Could you check a few things on this model? Use its own coordinates, in mm. A direction names the side the tool comes from. Round coordinates to 2 decimals unless told otherwise and drop trailing zeros. Loops run counter-clockwise (first coordinate to the right, second up) from the corner with the lowest first, then second, coordinate; pieces in that order, holes last. Notation, with made-up numbers: M 5,67.25 L 32,67.25 A22 cw 32,76.25 Z; hole C 82,-2.5 d6. An arc over 180 degrees is marked long. Answer in a Markdown table with one row per item.
```python
from build123d import *

# Parameters (mm, degrees)
SKETCH3_W           = 70
SKETCH3_H           = 70
BOSS_EXTRUDE1_DEPTH = 2.105
SKETCH6_R           = 3
SKETCH6_W           = 30
SKETCH6_H           = 30
CUT_EXTRUDE5_DEPTH  = 2.105
CUT_EXTRUDE7_DEPTH  = 0.2
FILLET1_R           = 3


with BuildPart() as part:
    # Sketch3 → Boss-Extrude1 (new body)
    with BuildSketch(Plane.XY):
        Rectangle(SKETCH3_W, SKETCH3_H)
    extrude(amount=BOSS_EXTRUDE1_DEPTH)

    # Sketch6 → Cut-Extrude5 (cut)
    with BuildSketch(Plane.XY.offset(2.105)):
        with Locations((0, 25)):
            Circle(SKETCH6_R)
        with Locations((25, 25)):
            Circle(SKETCH6_R)
        with Locations((25, 0)):
            Circle(SKETCH6_R)
        with Locations((25, -25)):
            Circle(SKETCH6_R)
        with Locations((0, -25)):
            Circle(SKETCH6_R)
        with Locations((-25, -25)):
            Circle(SKETCH6_R)
        with Locations((-25, 0)):
            Circle(SKETCH6_R)
        with Locations((-25, 25)):
            Circle(SKETCH6_R)
        Rectangle(SKETCH6_W, SKETCH6_H)
    extrude(amount=-CUT_EXTRUDE5_DEPTH, mode=Mode.SUBTRACT)

    # Sketch8 → Cut-Extrude7 (cut)
    with BuildSketch(Plane.XY.offset(2.105)):
        with BuildLine():
            Line((15, 5), (15, 15))
            Line((15, 15), (20.732380758, 13.932380758))
            ThreePointArc((20.732380758, 13.932380758), (24, 10), (20.732380758, 6.067619242))
            Line((20.732380758, 6.067619242), (15, 5))
        make_face()
        with BuildLine():
            Line((-15, -15), (-20.732380758, -13.932380758))
            ThreePointArc((-20.732380758, -13.932380758), (-24, -10), (-20.732380758, -6.067619242))
            Line((-20.732380758, -6.067619242), (-15, -5))
            Line((-15, -5), (-15, -15))
        make_face()
    extrude(amount=-CUT_EXTRUDE7_DEPTH, mode=Mode.SUBTRACT)

    # Fillet1
    fillet1_edges = [part.edges().sort_by_distance(p)[0] for p in [
        (35, -35, 1.0525),
        (-35, -35, 1.0525),
        (-35, 35, 1.0525),
        (35, 35, 1.0525),
    ]]
    fillet(fillet1_edges, radius=FILLET1_R)


solid = part.part
```
1) If we mould it in two halves opening along Y, with no side actions, what happens to faces 4 (the face through (34.1, -34.14, 1.07)), 5 (the face through (34.1, 34.14, 1.07)), 6 (the face through (22, 0, 1)), 7 (the face through (-0.65, -27.93, 1.07))? For each: released by +Y, released by -Y, zero draft, split by the parting line, or undercut.
Computed:
| item | result |
|---|---|
| face 4 | released by -Y |
| face 5 | released by +Y |
| face 6 | undercut |
| face 7 | undercut |
2) I want a section at A-A, the plane x = -25. Please give me the cut outline in (y, z) (3 decimals), plus the area to 3 significant figures.
Computed:
| item | result |
|---|---|
| outline | M -35,0 L -28,0 L -28,2.105 L -35,2.105 Z; M -22,0 L -3,0 L -3,2.105 L -22,2.105 Z; M 3,0 L 22,0 L 22,2.105 L 3,2.105 Z; M 28,0 L 35,0 L 35,2.105 L 28,2.105 Z |
| area | 109 mm² |
3) I want a section at D-D, the plane z = 0.7. State how many separate pieces and enclosed holes the cut face has, plus the area to 3 significant figures.
Computed:
| item | result |
|---|---|
| separate pieces | 1 |
| enclosed holes | 9 |
| area | 3,770 mm² |
4) I need wall thicknesses on line 1 (Y direction, x = 25, z = 0.75); line 2 (Y direction, x = 0, z = 1.3); line 3 (Y direction, x = -7, z = 1.2). Which ranges of each line are inside material? Lowest first, please.
Computed:
| item | result |
|---|---|
| line 1 | y = -35 to -28, -22 to -3, 3 to 22, 28 to 35 |
| line 2 | y = -35 to -28, -22 to -15, 15 to 22, 28 to 35 |
| line 3 | y = -35 to -15, 15 to 35 |
5) Will this pin go through, and if not, where does the flat tip stop? P1, Ø4.5, axis at x = 17.5, y = 12, coming from the +Z side (3 decimals).
Computed:
| item | result |
|---|---|
| P1 | stops at z = 1.905 |
6) Which directions (+Z, -Z, +X, -X, +Y, -Y) give clear straight access to the entire face, cutting with the end or side of a thin tool? Please do faces 1 (the face through (0, 16, 0)), 2 (the face through (-15, 0, 1)), 3 (the face through (-18, -10, 1.905)).
Computed:
| item | result |
|---|---|
| face 1 | -Z, +X, -X, +Y, -Y |
| face 2 | +Z, -Z |
| face 3 | +Z |
7) I want a section at C-C, the plane x = -8.5. Please give me the cut outline in (y, z) (3 decimals).
Computed:
| item | result |
|---|---|
| outline | M -35,0 L -15,0 L -15,2.105 L -35,2.105 Z; M 15,0 L 35,0 L 35,2.105 L 15,2.105 Z |
